For this review, take the finished solid that the model builds, in its own axes (mm). Face numbers are marked on the shaded views. A direction names the side the tool comes from. Round coordinates to 2 decimals unless told otherwise and drop trailing zeros. Write each loop counter-clockwise with the first axis right and the second up, starting at its lowest first coordinate (ties: lowest second). Pieces come first, ordered by that corner, then holes. Notation, with made-up numbers: M 62,47 L 69,47 A30 cw 69,84 Z; hole C 82,48 d2. An arc over 180 degrees is marked long. Use one line per item in the form item = value. Start each with the question number.
Item 1: Draft analysis for pull direction Y (two halves, no side actions). For the marked faces 3, 4 and 5, state which applies: released by +Y, released by -Y, zero draft, split by the parting line, or undercut.
Item 2: Add section B-B (y = 0). State the section outline as (x, z) points.
Item 3: Add section C-C (z = -2). State the section outline as (x, y) points, and give its area (3 significant figures).
Item 4: For P1, Ø1, axis at x = 1, z = 4, coming from the -Y side; P2, Ø1, axis at y = 0, z = 1, coming from the -X side; P3, Ø0.7, axis at x = -0.5, y = 0, coming from the +Z side, all flat-tipped, find the tip position at first contact; note any pin that passes through.
Item 5: Add section A-A (z = 5). State the section outline as (x, y) points.
Item 6: For line 1 (Y direction, x = -0.1, z = 3.5); line 2 (Z direction, x = 0.4, y = 0.6); line 3 (Z direction, x = -1.55, y = 0.7), list the stretches that pass through material, from the lowest coordinate up. Write a range as [from, to].
Item 7: For the marked faces 1 and 2, list the 3-axis set-ups (+Z, -Z, +X, -X, +Y, -Y) from which the entire face can be reached by the end or side of a thin tool; tool diameter is ignored.
from build123d import *

# Parameters (mm, degrees)
CUT_EXTRUDE1_DEPTH = 1.7859375
CHAMFER1_SIZE      = 0.23241
CHAMFER2_SIZE      = 0.116205


with BuildPart() as part:
    # Sketch2 → Revolve1 (revolve)
    with BuildSketch(Plane(origin=(0, 0, 0), x_dir=(0, 0, -1), z_dir=(1, 0, 0)), mode=Mode.PRIVATE) as revolve1_sk:
        Polygon((6.1849, 0.94615), (5.70865, 1.4224), (-3.3401, 1.4224), (-3.3401, 2.3241), (-6.1849, 2.3241), (-6.1849, 0), (6.1849, 0), align=None)
    revolve(revolve1_sk.sketch.rotate(Axis((0, 0, -6.1849), (0, 0, 1)), 90), axis=Axis((0, 0, -6.1849), (0, 0, 1)))

    # Sketch4 → Cut-Extrude1 (cut)
    with BuildSketch(Plane.XY.offset(6.1849)):
        Polygon((0, 1.374815329), (-1.190625, 0.687407664), (-1.190625, -0.687407664), (0, -1.374815329), (1.190625, -0.687407664), (1.190625, 0.687407664), align=None)
    extrude(amount=-CUT_EXTRUDE1_DEPTH, mode=Mode.SUBTRACT)

    # Cut-Extrude2 cone 1 section (on through the dimple's axis) → Cut-Extrude2 (revolve, cut)
    with BuildSketch(Plane(origin=(0, 0, 6.1849), x_dir=(0, -1, 0), z_dir=(1, 0, 0))):
        Polygon((0, 0), (1.374815329, 0), (0, 0.79375), align=None)
    revolve(axis=Axis((0, 0, 6.1849), (0, 0, -1)), mode=Mode.SUBTRACT)

    # Chamfer1
    chamfer1_edges = [part.edges().sort_by_distance(p)[0] for p in [
        (2.3241, 0, 6.1849),
    ]]
    chamfer(chamfer1_edges, length=CHAMFER1_SIZE)

    # Chamfer2
    chamfer2_edges = [part.edges().sort_by_distance(p)[0] for p in [
        (2.3241, 0, 3.3401),
    ]]
    chamfer(chamfer2_edges, length=CHAMFER2_SIZE)


solid = part.part
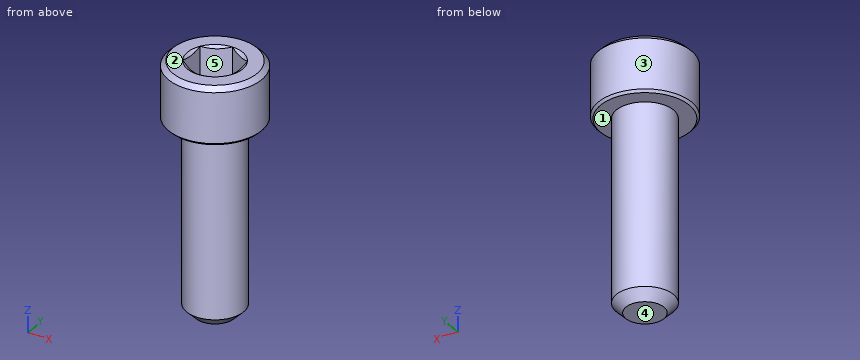
Calculated:
q1.face_3 = split by the parting line
q1.face_4 = zero draft
q1.face_5 = undercut
q2.outline = M -2.32,3.46 L -2.21,3.34 L -1.42,3.34 L -1.42,-5.71 L -0.95,-6.18 L 0.95,-6.18 L 1.42,-5.71 L 1.42,3.34 L 2.21,3.34 L 2.32,3.46 L 2.32,5.95 L 2.09,6.18 L 1.37,6.18 L 1.19,6.08 L 1.19,4.4 L -1.19,4.4 L -1.19,6.08 L -1.37,6.18 L -2.09,6.18 L -2.32,5.95 Z
q3.outline = C 0,0 d2.84
q3.area = 6.36 mm^2
q4.P1 = -2.27
q4.P2 = -1.42
q4.P3 = 4.4
q5.outline = C 0,0 d4.65; hole M -1.19,-0.69 L 0,-1.37 L 1.19,-0.69 L 1.19,0.69 L 0,1.37 L -1.19,0.69 Z
q6.line_1 = [-2.32, 2.32]
q6.line_2 = [-6.18, 4.4]
q6.line_3 = [3.34, 6.18]
q7.face_1 = -Z
q7.face_2 = +Z, +X, -X, +Y, -Y
